Study the drawing (mm; zero at the part's minimum x, y, z) and answer. Round coordinates to 2 decimals unless told otherwise and drop trailing zeros. Write each loop counter-clockwise with the first axis right and the second up, starting at its lowest first coordinate (ties: lowest second). Pieces come first, ordered by that corner, then holes. Notation, with made-up numbers: (-17.5, 16) -> (-3.5, 16) arc R22 ccw to (-3.5, 49) -> close; hole circle Ø2 at (-5.5, -10.75). An arc over 180 degrees is marked (long way). One line per question, with ' | ' between items. Start each with the question number.
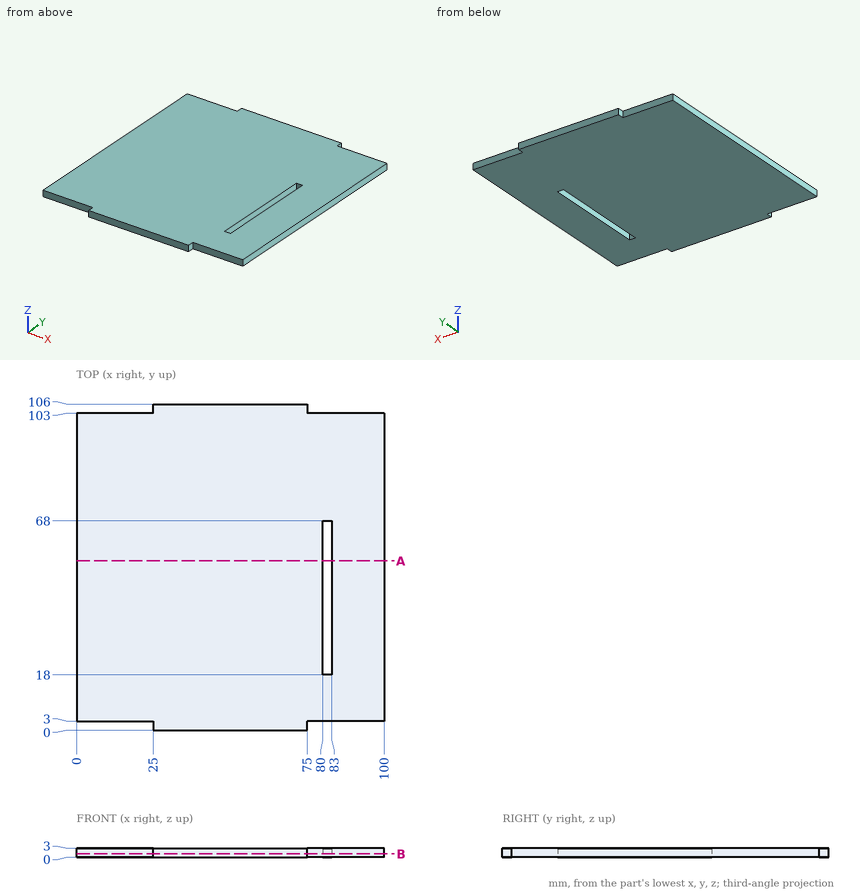
(1) A cutting plane is placed at A-A, the plane y = 55. Determine the outline of the cut face in (x, z), then the cut area to 3 significant figures.
(2) Consider L1, parallel to X at y = 45, z = 0.25; L2, parallel to Y at x = 14, z = 0.7. Determine where each line is inside the solid, lowest interval first.
(3) Given pin 1 Ø0.9 at (x, z) = (82, 1) entering from -Y; pin 2 Ø1.5 at (y, z) = (2, 2) entering from -X; pin 3 Ø1.5 at (x, z) = (81.5, 1) entering from +Y, each flat-ended and moving along its own axis, determine where each tip first touches the part or whether it passes through.
(4) A cutting plane is placed at B-B, the plane z = 1.2. Determine the outline of the cut face in (x, y), then the cut area to 4 significant figures.
Returned:
1) outline: (0, 0) -> (80, 0) -> (80, 3) -> (0, 3) -> close; (83, 0) -> (100, 0) -> (100, 3) -> (83, 3) -> close | area: 291 mm2
2) L1: 0 to 80, 83 to 100 | L2: 3 to 103
3) pin 1: y = 3 | pin 2: x = 25 | pin 3: y = 103
4) outline: (0, 3) -> (25, 3) -> (25, 0) -> (75, 0) -> (75, 3) -> (100, 3) -> (100, 103) -> (75, 103) -> (75, 106) -> (25, 106) -> (25, 103) -> (0, 103) -> close; hole (80, 18) -> (83, 18) -> (83, 68) -> (80, 68) -> close | area: 10,150 mm2
